```python
from build123d import *

# Parameters (mm, degrees)
BOSS_EXTRUDE1_DEPTH = 70
CUT_EXTRUDE1_DEPTH  = 1951.170505366
CUT_EXTRUDE2_DEPTH  = 32.5


with BuildPart() as part:
    # Sketch1 → Boss-Extrude1 (new body)
    with BuildSketch(Plane.XY):
        with BuildLine():
            Line((100, 0), (519, 0))
            ThreePointArc((519, 0), (589.710678119, 29.289321881), (619, 100))
            Line((619, 100), (619, 1748))
            ThreePointArc((619, 1748), (589.710678119, 1818.710678119), (519, 1848))
            Line((519, 1848), (100, 1848))
            ThreePointArc((100, 1848), (29.289321881, 1818.710678119), (0, 1748))
            Line((0, 1748), (0, 100))
            ThreePointArc((0, 100), (29.289321881, 29.289321881), (100, 0))
        make_face()
    extrude(amount=BOSS_EXTRUDE1_DEPTH)

    # Sketch2 → Cut-Extrude1 (cut, through all)
    with BuildSketch(Plane.ZY):
        with BuildLine():
            Line((70, 1848), (32, 1848))
            Line((32, 1848), (32, 127.446930132))
            ThreePointArc((32, 127.446930132), (41.702246447, 60.951215984), (70, 0))
            Line((70, 0), (70, 1848))
        make_face()
        with BuildLine():
            Line((0, 0), (32.698538924, 0))
            ThreePointArc((32.698538924, 0), (8.304907254, 61.659555872), (0, 127.446930132))
            Line((0, 127.446930132), (0, 0))
        make_face()
    extrude(amount=-CUT_EXTRUDE1_DEPTH, mode=Mode.SUBTRACT)

    # Sketch4 → Cut-Extrude2 (cut)
    with BuildSketch(Plane.ZY):
        with BuildLine():
            Line((1, 1848), (32, 1848))
            Line((32, 1848), (32, 127.446930132))
            ThreePointArc((32, 127.446930132), (41.702246447, 60.951215984), (70, 0))
            Line((70, 0), (33.840121275, 0))
            ThreePointArc((33.840121275, 0), (9.341966472, 61.641927348), (1, 127.446930132))
            Line((1, 127.446930132), (1, 1848))
        make_face()
    extrude(amount=-CUT_EXTRUDE2_DEPTH, mode=Mode.SUBTRACT)


solid = part.part
```
CAD build for the part. Positions are in the model's coordinates, mm. A direction names the side the tool comes from. Coordinates: 2 decimals unless noted, no trailing zeros. Write each loop counter-clockwise with the first axis right and the second up, starting at its lowest first coordinate (ties: lowest second). Pieces come first, ordered by that corner, then holes. Notation, with made-up numbers: (41, -34) -> (77, -34) arc R12 cw to (77, -25) -> close; hole circle Ø4 at (27, 17). An arc over 180 degrees is marked (long way). Use CSV: the item, a comma, the result in double quotes. Start each with the question number.
Item 1: Band-saw the part on B-B, the plane y = 926. Write the cut outline in (x, z), plus the area to 3 significant figures.
Item 2: Drop flat-ended pins along their axis: P1, Ø16.5, axis at y = 1205, z = 33.5, coming from the -X side; P2, Ø12, axis at x = 457.5, y = 1581.5, coming from the +Z side; P3, Ø2, axis at x = 112.5, z = 20.5, coming from the -Y side. Give the stop position or say it passes through.
Item 3: Band-saw the part on A-A, the plane x = 265. Write the cut outline in (y, z), plus the area to 3 significant figures.
Item 4: Wall check: probe 1 along Z at (x, y) = (164, 1215); probe 2 along X at (y, z) = (1112, 11); probe 3 along Y at (x, z) = (39.5, 24). Give the ranges that are in metal, low to high.
Item 5: Tool access for faces 1 (the flat face through (305, 1000, 0)), 2 (the cylindrical face through (19.6, 86.5, 4.2)), 3 (the flat face through (322, 1000, 32)): list every direction of +Z, -Z, +X, -X, +Y, -Y with a clear straight run to the whole face (end or side of a thin tool).
Response values:
1,outline,"(0, 0) -> (619, 0) -> (619, 32) -> (32.5, 32) -> (32.5, 1) -> (0, 1) -> close"
1,area,"18,800 mm2"
2,P1,"stops at x = 32.5"
2,P2,"stops at z = 32"
2,P3,"stops at y = 22.94"
3,outline,"(0, 32.7) arc R264.72 ccw to (127.45, 0) -> (1848, 0) -> (1848, 32) -> (127.45, 32) arc R232.72 cw to (0, 70) -> close"
3,area,"59,300 mm2"
4,probe 1,"z = 0 to 32"
4,probe 2,"x = 32.5 to 619"
4,probe 3,"y = 20.38 to 1827.62"
5,face 1,"-Z, +X, -X, +Y, -Y"
5,face 2,"+Z, -X, +Y"
5,face 3,"+Z, +X, -X, +Y"
